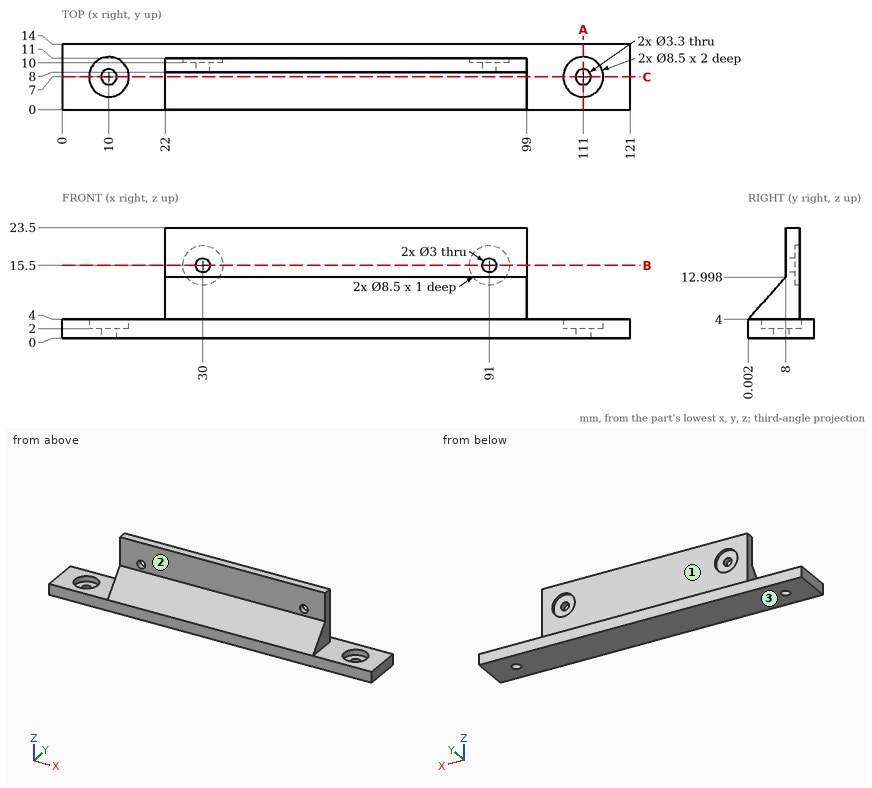
Geometry check sheet. Reference: drawing and pictorial views, mm from the part's lowest x, y, z. A direction names the side the tool comes from. Coordinates: 2 decimals unless noted, no trailing zeros. Order: outer loops, then holes, each group sorted by start corner. A loop starts at its lowest first (then second) coordinate and runs counter-clockwise, first axis right, second up. Notation, with made-up numbers: (-27, 9) -> (-15, 9) arc R20 ccw to (-15, 45) -> close; hole circle Ø5 at (22, -26.75). An arc over 180 degrees is marked (long way). Use CSV: the item, a comma, the result in double quotes. Start each with the question number.
Q1. Section check A-A, the plane x = 111. Record the cut outline in (y, z).
Q2. Section check B-B, the plane z = 15.5. Record the cut outline in (x, y), and give its area (3 significant figures).
Q3. Section check C-C, the plane y = 7. Record the cut outline in (x, z), and give its area (3 significant figures).
Q4. Tool access check on the marked faces 1, 2 and 3. Record the directions out of +Z, -Z, +X, -X, +Y, -Y that give a thin tool (end or side, any length) a straight path to the whole face; none if there is none.
Q5. Thickness scan on line 1 along X through (y, z) = (10.35, 15.5); line 2 along X through (y, z) = (9.55, 15.5); line 3 along Y through (x, z) = (10, 3.4). Record the ranges inside material, lowest first.
Q6. Depth check by flat-ended pin: P1, Ø8, axis at y = 12.5, z = 4, coming from the -X side; P2, Ø3, axis at y = 11, z = 12, coming from the -X side; P3, Ø13.5, axis at x = 30, z = 15.5, coming from the +Y side; P4, Ø4, axis at x = 110, y = 7.5, coming from the +Z side. Enter the tip coordinate at first touch or a pass-through.
Returned:
1,outline,"(0, 0) -> (5.35, 0) -> (5.35, 2) -> (2.75, 2) -> (2.75, 4) -> (0, 4) -> close; (8.65, 0) -> (14, 0) -> (14, 4) -> (11.25, 4) -> (11.25, 2) -> (8.65, 2) -> close"
2,outline,"(22, 8) -> (28.5, 8) -> (28.5, 10) -> (25.75, 10) -> (25.75, 11) -> (22, 11) -> close; (31.5, 8) -> (89.5, 8) -> (89.5, 10) -> (86.75, 10) -> (86.75, 11) -> (34.25, 11) -> (34.25, 10) -> (31.5, 10) -> close; (92.5, 8) -> (99, 8) -> (99, 11) -> (95.25, 11) -> (95.25, 10) -> (92.5, 10) -> close"
2,area,"202 mm^2"
3,outline,"(0, 0) -> (8.35, 0) -> (8.35, 2) -> (5.75, 2) -> (5.75, 4) -> (0, 4) -> close; (11.65, 0) -> (109.35, 0) -> (109.35, 2) -> (106.75, 2) -> (106.75, 4) -> (99, 4) -> (99, 11.87) -> (22, 11.87) -> (22, 4) -> (14.25, 4) -> (14.25, 2) -> (11.65, 2) -> close; (112.65, 0) -> (121, 0) -> (121, 4) -> (115.25, 4) -> (115.25, 2) -> (112.65, 2) -> close"
3,area,"1,040 mm^2"
4,face 1,"+Z, +X, -X, +Y"
4,face 2,"+Z, +X, -X, -Y"
4,face 3,"-Z, +X, -X, +Y, -Y"
5,line 1,"x = 22 to 25.75, 34.25 to 86.75, 95.25 to 99"
5,line 2,"x = 22 to 28.5, 31.5 to 89.5, 92.5 to 99"
5,line 3,"y = 0 to 2.75, 11.25 to 14"
6,P1,"stops at x = 0"
6,P2,"stops at x = 22"
6,P3,"stops at y = 11"
6,P4,"stops at z = 2"
